```python
from build123d import *

# Parameters (mm, degrees)
F0_R     = 2.5
F1_DEPTH = 2.5


with BuildPart() as f1:
    # F0 (on Front) → F1 (new body)
    with BuildSketch(Plane.XZ):
        with BuildLine():
            Line((-39.0163958073, 32.069671154), (-39.0163958073, -17.930328846))
            Line((-39.0163958073, -17.930328846), (40.9836041927, -17.930328846))
            Line((40.9836041927, -17.930328846), (40.9836041927, 32.069671154))
            Line((40.9836041927, 32.069671154), (20.9836041927, 32.069671154))
            ThreePointArc((20.9836041927, 32.069671154), (0.9836041927, 51.7268625575), (-19.0163958073, 32.069671154))
            Line((-19.0163958073, 32.069671154), (-39.0163958073, 32.069671154))
        make_face()
        with BuildLine():
            Line((-32.4271805924, 11.4579676845), (-32.4271805924, 26.6955864939))
            Line((-32.4271805924, 26.6955864939), (-28.121694516, 26.6955864939))
            add(Edge.make_bspline(
                [(-28.121694516, 26.6955864939), (-25.0901787581, 26.6955864939), (-23.7345009192, 25.7884662672)],
                knots=[0, 0, 0, 1, 1, 1], degree=2))
            add(Edge.make_bspline(
                [(-23.7345009192, 25.7884662672), (-22.3788230803, 24.8813460404), (-22.3788230803, 22.923700551)],
                knots=[0, 0, 0, 1, 1, 1], degree=2))
            add(Edge.make_bspline(
                [(-22.3788230803, 22.923700551), (-22.3788230803, 21.5663552116), (-23.1342007691, 20.6859149915)],
                knots=[0, 0, 0, 1, 1, 1], degree=2))
            add(Edge.make_bspline(
                [(-23.1342007691, 20.6859149915), (-23.889578458, 19.8054747714), (-25.3403038207, 19.5453447064)],
                knots=[0, 0, 0, 1, 1, 1], degree=2))
            Line((-25.3403038207, 19.5453447064), (-25.3403038207, 19.4419596805))
            add(Edge.make_bspline(
                [(-25.3403038207, 19.4419596805), (-21.8685679527, 18.8483295321), (-21.8685679527, 15.7934687684)],
                knots=[0, 0, 0, 1, 1, 1], degree=2))
            add(Edge.make_bspline(
                [(-21.8685679527, 15.7934687684), (-21.8685679527, 13.7524482582), (-23.2492582979, 12.6052079713)],
                knots=[0, 0, 0, 1, 1, 1], degree=2))
            add(Edge.make_bspline(
                [(-23.2492582979, 12.6052079713), (-24.6299486431, 11.4579676845), (-27.1111892634, 11.4579676845)],
                knots=[0, 0, 0, 1, 1, 1], degree=2))
            Line((-27.1111892634, 11.4579676845), (-32.4271805924, 11.4579676845))
        make_face(mode=Mode.SUBTRACT)
        with BuildLine():
            add(Edge.make_bspline(
                [(-10.4111725884, 21.4946526937), (-8.9987997353, 19.8988547948), (-8.9987997353, 17.1808291152)],
                knots=[0, 0, 0, 1, 1, 1], degree=2))
            add(Edge.make_bspline(
                [(-8.9987997353, 17.1808291152), (-8.9987997353, 14.3860984166), (-10.4045025867, 12.8169805243)],
                knots=[0, 0, 0, 1, 1, 1], degree=2))
            add(Edge.make_bspline(
                [(-10.4045025867, 12.8169805243), (-11.8102054381, 11.247862632), (-14.2914460585, 11.247862632)],
                knots=[0, 0, 0, 1, 1, 1], degree=2))
            add(Edge.make_bspline(
                [(-14.2914460585, 11.247862632), (-15.825546442, 11.247862632), (-17.0128067388, 11.9682228121)],
                knots=[0, 0, 0, 1, 1, 1], degree=2))
            add(Edge.make_bspline(
                [(-17.0128067388, 11.9682228121), (-18.2000670356, 12.6885829922), (-18.8470571974, 14.0325883282)],
                knots=[0, 0, 0, 1, 1, 1], degree=2))
            add(Edge.make_bspline(
                [(-18.8470571974, 14.0325883282), (-19.4940473591, 15.3765936642), (-19.4940473591, 17.1808291152)],
                knots=[0, 0, 0, 1, 1, 1], degree=2))
            add(Edge.make_bspline(
                [(-19.4940473591, 17.1808291152), (-19.4940473591, 19.9722248131), (-18.0966820098, 21.5313377029)],
                knots=[0, 0, 0, 1, 1, 1], degree=2))
            add(Edge.make_bspline(
                [(-18.0966820098, 21.5313377029), (-16.6993166604, 23.0904505927), (-14.2180760401, 23.0904505927)],
                knots=[0, 0, 0, 1, 1, 1], degree=2))
            add(Edge.make_bspline(
                [(-14.2180760401, 23.0904505927), (-11.8235454415, 23.0904505927), (-10.4111725884, 21.4946526937)],
                knots=[0, 0, 0, 1, 1, 1], degree=2))
        make_face(mode=Mode.SUBTRACT)
        with BuildLine():
            add(Edge.make_bspline(
                [(-4.2330835439, 21.3595851599), (-3.025813242, 23.0671055868), (-0.6479576476, 23.0671055868)],
                knots=[0, 0, 0, 1, 1, 1], degree=2))
            add(Edge.make_bspline(
                [(-0.6479576476, 23.0671055868), (1.6031679152, 23.0671055868), (2.8487907266, 21.5296702025)],
                knots=[0, 0, 0, 1, 1, 1], degree=2))
            add(Edge.make_bspline(
                [(2.8487907266, 21.5296702025), (4.094413538, 19.9922348181), (4.094413538, 17.1808291152)],
                knots=[0, 0, 0, 1, 1, 1], degree=2))
            add(Edge.make_bspline(
                [(4.094413538, 17.1808291152), (4.094413538, 14.3660884116), (2.8387857241, 12.8069755218)],
                knots=[0, 0, 0, 1, 1, 1], degree=2))
            add(Edge.make_bspline(
                [(2.8387857241, 12.8069755218), (1.5831579102, 11.247862632), (-0.6479576476, 11.247862632)],
                knots=[0, 0, 0, 1, 1, 1], degree=2))
            add(Edge.make_bspline(
                [(-0.6479576476, 11.247862632), (-1.7651829269, 11.247862632), (-2.6873106574, 11.659735235)],
                knots=[0, 0, 0, 1, 1, 1], degree=2))
            add(Edge.make_bspline(
                [(-2.6873106574, 11.659735235), (-3.6094383879, 12.0716078379), (-4.2330835439, 12.9287030522)],
                knots=[0, 0, 0, 1, 1, 1], degree=2))
            Line((-4.2330835439, 12.9287030522), (-4.3598135755, 12.9287030522))
            Line((-4.3598135755, 12.9287030522), (-4.7233286664, 11.4579676845))
            Line((-4.7233286664, 11.4579676845), (-5.9639489766, 11.4579676845))
            Line((-5.9639489766, 11.4579676845), (-5.9639489766, 27.6760767391))
            Line((-5.9639489766, 27.6760767391), (-4.2330835439, 27.6760767391))
            Line((-4.2330835439, 27.6760767391), (-4.2330835439, 23.7341057536))
            add(Edge.make_bspline(
                [(-4.2330835439, 23.7341057536), (-4.2330835439, 22.4101104226), (-4.3164585647, 21.3595851599)],
                knots=[0, 0, 0, 1, 1, 1], degree=2))
            Line((-4.3164585647, 21.3595851599), (-4.2330835439, 21.3595851599))
        make_face(mode=Mode.SUBTRACT)
        with Locations((0.9836041927, 40.6512729824)):
            Circle(F0_R, mode=Mode.SUBTRACT)
    extrude(amount=F1_DEPTH)


solid = f1.part
```
Work out the finished part from the listing and answer in its coordinate system (mm). A direction names the side the tool comes from. Give positions to 0.01 mm unless a question says otherwise; leave off trailing zeros. Order: outer loops, then holes, each group sorted by start corner. A loop starts at its lowest first (then second) coordinate and runs counter-clockwise, first axis right, second up.
1. Each of these flat-tipped pins is pushed along its axis until it touches: P1, Ø1.2, axis at x = -30, y = -1.5, coming from the +Z side; P2, Ø0.6, axis at x = -5.5, y = -2, coming from the +Z side; P3, Ø1.5, axis at y = -2, z = 44, coming from the -X side. Where does it stop, or does it pass through?
Result sheet:
P1: stops at z = 32.07
P2: stops at z = 50.75
P3: stops at x = -15.36
2. Section A-A, the plane x = 22.5 is taken. Determine the outline of the cut face in (y, z), and give its area (3 significant figures).
Result sheet:
outline: (-2.5, -17.93) - (0, -17.93) - (0, 32.07) - (-2.5, 32.07) - close
area: 125 mm2
3. For faces 1 (the cylindrical face through (1.419, -1.232, 51.722)), 2 (the flat face through (-5.964, -1, 19)), 3 (the flat face through (-29, -1, 32.07)), 4 (the flat face through (31, -1, 32.07)), determine the directions among +Z, -Z, +X, -X, +Y, -Y from which every point of the face is accessible in a straight line to the end or side of a thin tool.
Result sheet:
face 1: +Z, +Y, -Y
face 2: +Y, -Y
face 3: +Z, -X, +Y, -Y
face 4: +Z, +X, +Y, -Y
4. Section B-B, the plane y = -2.05 is taken. Give the number of separate pieces and of enclosed holes in the cut face, and give its area (3 significant figures).
Result sheet:
separate pieces: 1
enclosed holes: 4
area: 4,240 mm2
5. Section C-C, the plane z = 47 is taken. Determine the outline of the cut face in (x, y).
Result sheet:
outline: (-11.93, -2.5) - (13.9, -2.5) - (13.9, 0) - (-11.93, 0) - close
6. Straight lines are drawn through the part: L1, parallel to Z at x = -30, y = -1.05; L2, parallel to Z at x = -1, y = -2; L3, parallel to X at y = -0.65, z = 22. For each, find the intervals that lie inside material, in ascending order.
Result sheet:
L1: z = -17.93 to 11.46, 26.7 to 32.07
L2: z = -17.93 to 11.26, 23.06 to 39.13, 42.17 to 51.63
L3: x = -39.02 to -32.43, -22.48 to -17.61, -10.93 to -5.96, -4.27 to -3.68, 2.41 to 40.98
